Could you check a few things on this drawing? It's one solid part, dimensions in mm from its lowest x, y, z. A direction names the side the tool comes from. Give positions to 0.01 mm unless a question says otherwise; leave off trailing zeros. Loops run counter-clockwise (first coordinate to the right, second up) from the corner with the lowest first, then second, coordinate; pieces in that order, holes last. Notation, with made-up numbers: M 86,-37 L 123,-37 A30 cw 123,-10 Z; hole C -4.5,22 d5. An arc over 180 degrees is marked long. Write each question's results on one line, items separated by ' | '. Start each with the question number.
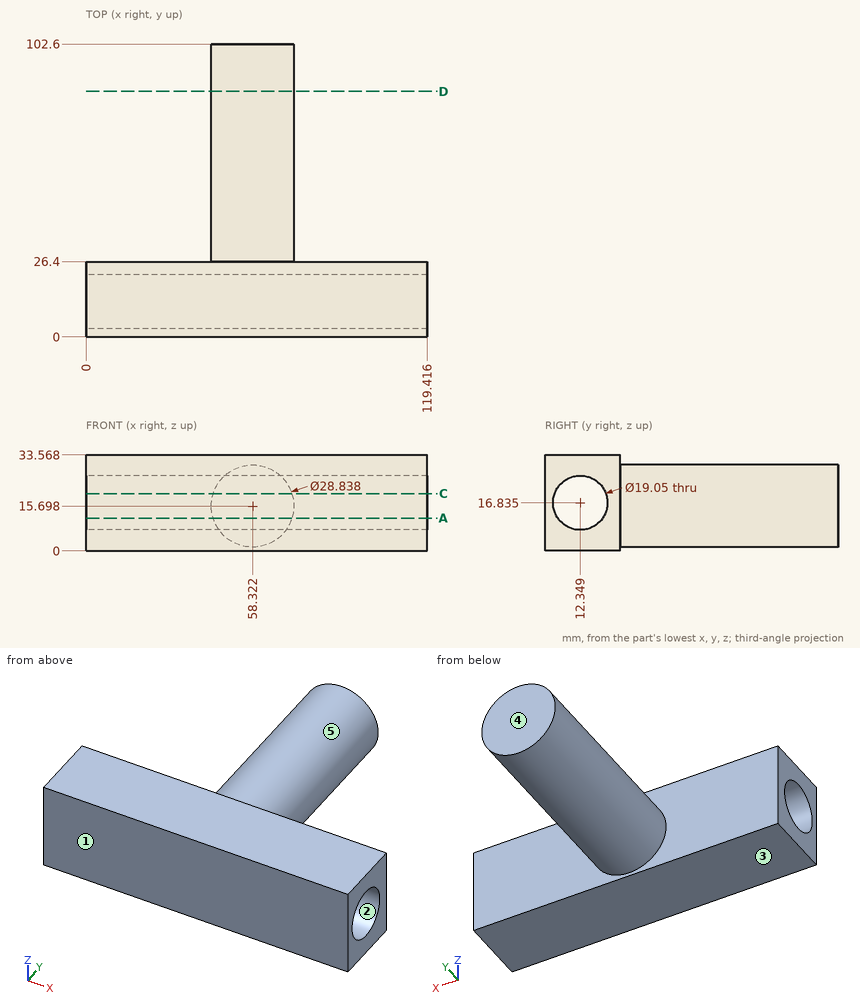
1) If we section it at A-A on z = 11.5: Write out the boundary of the cut face in (x, y) (1 decimal), plus the area to 3 significant figures.
2) Which directions (+Z, -Z, +X, -X, +Y, -Y) give clear straight access to the entire face, cutting with the end or side of a thin tool? Please do the marked faces 4 and 5.
3) Please list where these lines run through material, in increasing order: line 1 (Z direction, x = 102, y = 12.5); line 2 (Y direction, x = 59, z = 31); line 3 (Y direction, x = 51, z = 24) (1 decimal). Write a range as from..to.
4) Thinking about a two-plate mould opening in Y: for the marked faces 1, 2 and 3, which applies, pulls with the +Y half, pulls with the -Y half, needs draft (parallel to the pull), parting line crosses it, or undercut?
5) If we section it at C-C on z = 20: Write out the boundary of the cut face in (x, y) (1 decimal), plus the area to 3 significant figures.
6) If we section it at D-D on y = 86: Write out the boundary of the cut face in (x, z).
7) I'm going to push flat-ended pins straight in: P1, Ø5, axis at y = 87, z = 24.5, coming from the -X side; P2, Ø3, axis at x = 77.5, z = 23, coming from the +Y side; P3, Ø5, axis at y = 55, z = 18, coming from the -X side. Where does each tip first touch, or does it pass through?
Calculated:
1) outline: M 0,0 L 119.4,0 L 119.4,4.5 L 0,4.5 Z; M 0,20.2 L 119.4,20.2 L 119.4,26.4 L 72.1,26.4 L 72.1,102.6 L 44.5,102.6 L 44.5,26.4 L 0,26.4 Z | area: 3,370 mm2
2) face 4: +Z, -Z, +X, -X, +Y | face 5: +Y
3) line 1: z = 0..7.31, 26.36..33.57 | line 2: y = 0..26.4 | line 3: y = 0..6.1, 18.6..102.6
4) face 1: pulls with the -Y half | face 2: undercut | face 3: needs draft
5) outline: M 0,0 L 119.4,0 L 119.4,3.4 L 0,3.4 Z; M 0,21.3 L 119.4,21.3 L 119.4,26.4 L 72.1,26.4 L 72.1,102.6 L 44.6,102.6 L 44.6,26.4 L 0,26.4 Z | area: 3,100 mm2
6) outline: C 58.32,15.7 d28.84
7) P1: stops at x = 45.35 | P2: stops at y = 26.4 | P3: stops at x = 43.9
